Geometry check sheet. Reference: the model listing, model coordinates, mm. A direction names the side the tool comes from. Round coordinates to 2 decimals unless told otherwise and drop trailing zeros. Write each loop counter-clockwise with the first axis right and the second up, starting at its lowest first coordinate (ties: lowest second). Pieces come first, ordered by that corner, then holes. Notation, with made-up numbers: (27.5, 58) -> (61.5, 58) arc R18 cw to (61.5, 91) -> close; hole circle Ø10 at (6.25, -10.75). An arc over 180 degrees is marked (long way). Use a Markdown table: item, result.
```python
from build123d import *

# Parameters (mm, degrees)
SKETCH1_R             = 31
BOSS_EXTRUDE1_DEPTH   = 15.6
SKETCH2_R             = 23.5
BOSS_EXTRUDE2_DEPTH   = 8.4
SKETCH3_R             = 12.875
CUT_EXTRUDE1_DEPTH    = 50.979995998
SKETCH4_R             = 26.625
CUT_EXTRUDE2_DEPTH    = 11
M6X1_0_TAPPED_HOLE1_D = 5
CIRPATTERN1_COUNT     = 3


with BuildPart() as part:
    # Sketch1 → Boss-Extrude1 (new body)
    with BuildSketch(Plane.XY):
        Circle(SKETCH1_R)
    extrude(amount=BOSS_EXTRUDE1_DEPTH)

    # Sketch2 → Boss-Extrude2 (add)
    with BuildSketch(Plane.XY.offset(15.6)):
        Circle(SKETCH2_R)
    extrude(amount=BOSS_EXTRUDE2_DEPTH)

    # Sketch3 → Cut-Extrude1 (cut, through all)
    with BuildSketch(Plane.XY.offset(24)):
        Circle(SKETCH3_R)
    extrude(amount=-CUT_EXTRUDE1_DEPTH, mode=Mode.SUBTRACT)

    # Sketch4 → Cut-Extrude2 (cut)
    with BuildSketch(Plane(origin=(0, 0, 0), x_dir=(-1, 0, 0), z_dir=(0, 0, -1))):
        Circle(SKETCH4_R)
    extrude(amount=-CUT_EXTRUDE2_DEPTH, mode=Mode.SUBTRACT)

    # M6x1.0 Tapped Hole1 (through all)
    with Locations(Plane.XY.offset(24)):
        with Locations((-5.7, 15.830054485), (5.7, 15.830054485)):
            m6x1_0_tapped_hole1 = Hole(M6X1_0_TAPPED_HOLE1_D / 2)

    # CirPattern1: M6x1.0 Tapped Hole1 ×3 about axis
    cirpattern1_axis = Axis((0, 0, 0), (0, 0, 1))
    for i in range(1, CIRPATTERN1_COUNT):
        add(m6x1_0_tapped_hole1.rotate(cirpattern1_axis, i * 360 / CIRPATTERN1_COUNT), mode=Mode.SUBTRACT)


solid = part.part
```
(1) Section check D-D on x = 25.5. Record the cut outline in (y, z), plus the area to 3 significant figures.
A:
| item | result |
|---|---|
| outline | (-17.63, 0) -> (-7.66, 0) -> (-7.66, 11) -> (7.66, 11) -> (7.66, 0) -> (17.63, 0) -> (17.63, 15.6) -> (-17.63, 15.6) -> close |
| area | 382 mm2 |
(2) Gauge pin test, flat ends, axial feed: pin 1 Ø1.5 at (y, z) = (21, 19.5) entering from -X; pin 2 Ø4.5 at (x, y) = (5.7, 15.83) entering from +Z; pin 3 Ø6 at (x, y) = (-16.56, -2.98) entering from -Z; pin 4 Ø4 at (x, z) = (-11, 5.5) entering from -Y. Record the tip position at first contact, or that the pin passes through.
A:
| item | result |
|---|---|
| pin 1 | stops at x = -11.92 |
| pin 2 | passes through |
| pin 3 | stops at z = 11 |
| pin 4 | stops at y = -29.66 |
(3) Access from +Z, -Z, +X, -X, +Y, -Y to the whole of each face (thin tool, end or side, straight path). Record for faces 1 (the face through (6.3, -11.5, 11)), 2 (the face through (10, -10, 24)).
A:
| item | result |
|---|---|
| face 1 | -Z |
| face 2 | +Z, +X, -X, +Y, -Y |
(4) Release check for a two-part mould opening along Y. For faces 3 (the face through (4.36, 17.94, 17.41)), 4 (the face through (22.4, 7.1, 19.7)), 5 (the face through (-14.06, -2.87, 17.41)), 6 (the face through (11, 21, 15.6)) record: +Y half, -Y half, draft (parallel to the pull), parting line (faces both ways), or undercut.
A:
| item | result |
|---|---|
| face 3 | undercut |
| face 4 | parting line |
| face 5 | undercut |
| face 6 | draft |
(5) Section check B-B on z = 7.75. Record the cut outline in (x, y) (3 decimals), plus the area to 3 significant figures.
A:
| item | result |
|---|---|
| outline | circle Ø62 at (0, 0); hole circle Ø53.25 at (0, 0) |
| area | 792 mm2 |
(6) Section check A-A on x = 0. Record the cut outline in (y, z) (3 decimals).
A:
| item | result |
|---|---|
| outline | (-31, 0) -> (-26.625, 0) -> (-26.625, 11) -> (-12.875, 11) -> (-12.875, 24) -> (-23.5, 24) -> (-23.5, 15.6) -> (-31, 15.6) -> close; (12.875, 11) -> (26.625, 11) -> (26.625, 0) -> (31, 0) -> (31, 15.6) -> (23.5, 15.6) -> (23.5, 24) -> (12.875, 24) -> close |
(7) Section check C-C on y = -9. Record the cut outline in (x, z), plus the area to 3 significant figures.
A:
| item | result |
|---|---|
| outline | (-29.66, 0) -> (-25.06, 0) -> (-25.06, 11) -> (-9.21, 11) -> (-9.21, 24) -> (-21.71, 24) -> (-21.71, 15.6) -> (-29.66, 15.6) -> close; (9.21, 11) -> (25.06, 11) -> (25.06, 0) -> (29.66, 0) -> (29.66, 15.6) -> (21.71, 15.6) -> (21.71, 24) -> (9.21, 24) -> close |
| area | 500 mm2 |
(8) Thickness scan on line 1 (X direction, y = -2.5, z = 12.75); line 2 (Y direction, x = 5.7, z = 17.25); line 3 (Y direction, x = 0, z = 3.5) (3 decimals). Record the ranges inside material, lowest first.
A:
| item | result |
|---|---|
| line 1 | x = -30.9 to -19.01, -14.11 to -12.63, 12.63 to 14.11, 19.01 to 30.9 |
| line 2 | y = -22.8 to -11.54, 11.54 to 13.33, 18.33 to 22.8 |
| line 3 | y = -31 to -26.625, 26.625 to 31 |
